For this review, take the finished solid that the model builds, in its own axes (mm). A direction names the side the tool comes from. Coordinates: 2 decimals unless noted, no trailing zeros. Loops run counter-clockwise (first coordinate to the right, second up) from the corner with the lowest first, then second, coordinate; pieces in that order, holes last. Notation, with made-up numbers: (78, 26) - (130, 26) arc R13 ccw to (130, 32) - close; hole circle Ø10 at (22.5, 52.25). An arc over 180 degrees is marked (long way). One line per item, written item: value. Start each with the question number.
1. Take a section at A-A, the plane z = 8.25. State the section outline as (x, y) points, and give its area (3 significant figures).
2. Insertion check: pin 1 (3.5 mm diameter, centred on x = -5, z = 8, fed in from -Y); pin 2 (6 mm diameter, centred on x = -9.5, z = 5.5, fed in from +Y); pin 3 (5 mm diameter, centred on y = 10.5, z = 10.5, fed in from -X); pin 4 (1.2 mm diameter, centred on x = -1, y = 10, fed in from +Z). Each pin has a flat end and moves straight along its axis. Give the tip position at first contact, or say it passes through.
3. Take a section at D-D, the plane y = 12.25. State the section outline as (x, z) points.
4. For faces 1 (the face through (-13.1, 10.78, 1.52)), 2 (the face through (-3, 11.35, 6)), 3 (the face through (-1.58, 8.43, 14.4)), 4 (the face through (-3.2, 13, 11)), list the 3-axis set-ups (+Z, -Z, +X, -X, +Y, -Y) from which the entire face can be reached by the end or side of a thin tool; tool diameter is ignored.
5. To check wall thickness, follow line 1 (X direction, y = 7.25, z = 1.25); line 2 (Y direction, x = -1.75, z = 7.75); line 3 (X direction, y = 13.5, z = 12.75). State the ranges of each line that lie inside material, in increasing order. Write a range as from..to.
6. Take a section at B-B, the plane y = 4.75. State the section outline as (x, z) points.
7. The part is to be moulded in two halves that separate along X. For faces 5 (the face through (-15.63, 13.46, 1.48)), 6 (the face through (0, 7, 7)), 7 (the face through (-14, 9, 3)), 8 (the face through (-13.7, 7, 1)), say which applies: released by +X, released by -X, zero draft, split by the parting line, or undercut.
```python
from build123d import *

# Parameters (mm, degrees)
F0_W        = 3.2
F0_H        = 9
F1_DEPTH    = 15
F0_H_2      = 3
F0_H_3      = 2.35
F2_DEPTH    = 3
F3_R        = 2
F4_R        = 1.99999
F5_T1_DEPTH = 3


# Not quite as in the source:
# - a fillet or chamfer that OpenCascade refuses, or shapes differently, is made with other operations: its cross-section is extruded or revolved along the edge and cut away or added
# - a fillet or chamfer is up to 0.001 mm smaller than in the source, because OpenCascade refuses the exact size


with BuildPart() as f1:
    # F0 (on Top) → F1 (new body)
    with BuildSketch(Plane.XY):
        with Locations((-1.6, 4.5)):
            Rectangle(F0_W, F0_H)
    extrude(amount=F1_DEPTH)



with BuildPart() as f1b:
    # F0 (on Top) → F1, piece 2 (new body)
    with BuildSketch(Plane.XY):
        with Locations((-1.6, 12.85)):
            Rectangle(F0_W, F0_H_2)
    extrude(amount=F1_DEPTH)


with BuildPart() as f1_1:
    add(f1.part)

    add(f1b.part)  # F2 merges F1b
    # F0 (on Top) → F2 (join)
    with BuildSketch(Plane.XY):
        with Locations((-1.6, 10.175)):
            Rectangle(F0_W, F0_H_3)
        with BuildLine():
            Line((-13.7, 11.35), (-3.2, 11.35))
            Line((-3.2, 11.35), (-3.2, 14.35))
            Line((-3.2, 14.35), (-13.7, 14.35))
            ThreePointArc((-13.7, 14.35), (-15.652562419, 13.4354686825), (-16.2, 11.35))
            Line((-16.2, 11.35), (-16.2, -0.65))
            Line((-16.2, -0.65), (-13.7, -0.65))
            Line((-13.7, -0.65), (-11.7, -0.65))
            Line((-11.7, -0.65), (-11.7, 1.85))
            Line((-11.7, 1.85), (-13.7, 1.85))
            Line((-13.7, 1.85), (-13.7, 11.35))
        make_face()
    extrude(amount=F2_DEPTH)

    # F3
    f3_edges = [f1_1.edges().sort_by_distance(p)[0] for p in [
        (-1.6, 9, 15),
    ]]
    fillet(f3_edges, radius=F3_R)

    # F4 (radius 2 in the source; OpenCascade refuses exactly that, so slightly less here)
    f4_edges = [f1_1.edges().sort_by_distance(p)[0] for p in [
        (-16.2, -0.65, 1.5),
        (-13.7, 11.35, 1.5),
        (-13.7, 1.85, 1.5),
    ]]
    fillet(f4_edges, radius=F4_R)

    # F5: fillet of radius 5 on 1 edges, made by hand

    # F5_s2 → F5_t1 (join)
    with BuildSketch(Plane.XZ.offset(-14.35)):
        with BuildLine():
            ThreePointArc((-8.2, 3), (-4.6644660941, 4.4644660941), (-3.2, 8))
            Line((-3.2, 8), (-3.2, 3))
            Line((-3.2, 3), (-8.2, 3))
        make_face()
    extrude(amount=F5_T1_DEPTH)


solid = f1_1.part
```
Solutions:
1. outline: (-3.2, 0) - (0, 0) - (0, 9) - (-3.2, 9) - close; (-3.2, 11.35) - (0, 11.35) - (0, 14.35) - (-3.2, 14.35) - close
1. area: 38.4 mm2
2. pin 1: through
2. pin 2: y = 14.35
2. pin 3: x = -3.2
2. pin 4: z = 3
3. outline: (-16.2, 0) - (0, 0) - (0, 15) - (-3.2, 15) - (-3.2, 8) arc R5 cw to (-8.2, 3) - (-16.2, 3) - close
4. face 1: +Z, -Z
4. face 2: +Z
4. face 3: +Z, +X, -X
4. face 4: +Z, -X, +Y, -Y
5. line 1: -16.2..-13.7, -3.2..0
5. line 2: 0..9, 11.35..14.35
5. line 3: -3.2..0
6. outline: (-16.2, 0) - (-13.7, 0) - (-13.7, 3) - (-16.2, 3) - close; (-3.2, 0) - (0, 0) - (0, 15) - (-3.2, 15) - close
7. face 5: released by -X
7. face 6: released by +X
7. face 7: zero draft
7. face 8: undercut
